```python
from build123d import *

# Parameters (mm, degrees)
CROQUIS1_W              = 41.18
CROQUIS1_H              = 12.95
CROQUIS1_R              = 1.5
SALIENTE_EXTRUIR1_DEPTH = 1
CROQUIS2_W              = 6
CROQUIS2_H              = 7.95
CORTAR_EXTRUIR1_DEPTH   = 0.5


with BuildPart() as part:
    # Croquis1 → Saliente-Extruir1 (new body)
    with BuildSketch(Plane.XY):
        with Locations((-20.59, 6.475)):
            Rectangle(CROQUIS1_W, CROQUIS1_H)
        with Locations((-38.68, 2.5)):
            Circle(CROQUIS1_R, mode=Mode.SUBTRACT)
        with Locations(Location((-38.68, 10.45, 0), (0, 0, 180))):
            Circle(CROQUIS1_R, mode=Mode.SUBTRACT)
        with Locations(Location((-2.5, 2.5, 0), (0, 0, 180))):
            Circle(CROQUIS1_R, mode=Mode.SUBTRACT)
        with Locations((-2.5, 10.45)):
            Circle(CROQUIS1_R, mode=Mode.SUBTRACT)
    extrude(amount=SALIENTE_EXTRUIR1_DEPTH)

    # Croquis2 → Cortar-Extruir1 (cut)
    with BuildSketch(Plane.XY.offset(1)):
        with Locations((-7.5, 6.475)):
            Rectangle(CROQUIS2_W, CROQUIS2_H)
    extrude(amount=-CORTAR_EXTRUIR1_DEPTH, mode=Mode.SUBTRACT)


solid = part.part
```
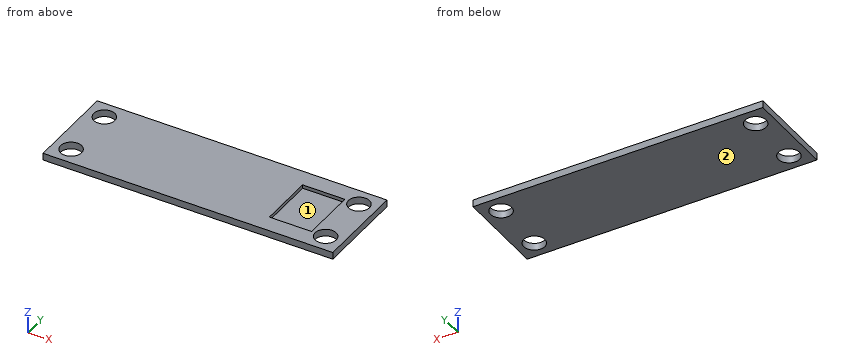
Source: CAD feature listing. Evaluate the final solid. Frame: model axes, mm. Face numbers are marked on the shaded views. Give positions to 0.01 mm unless a question says otherwise; leave off trailing zeros. Order: outer loops, then holes, each group sorted by start corner. A loop starts at its lowest first (then second) coordinate and runs counter-clockwise, first axis right, second up. Notation, with made-up numbers: (75.25, 80.5) -> (120.25, 80.5) arc R23 cw to (120.25, 115.5) -> close; hole circle Ø10 at (20.25, 4). An arc over 180 degrees is marked (long way). Use a Markdown table: item, result.
Q1. Section B-B (x = -2.5). Return the cut outline in (y, z).
A:
| item | result |
|---|---|
| outline | (0, 0) -> (1, 0) -> (1, 1) -> (0, 1) -> close; (4, 0) -> (8.95, 0) -> (8.95, 1) -> (4, 1) -> close; (11.95, 0) -> (12.95, 0) -> (12.95, 1) -> (11.95, 1) -> close |
Q2. Section C-C (y = 8.25). Return the cut outline in (x, z), and give its area (3 significant figures).
A:
| item | result |
|---|---|
| outline | (-41.18, 0) -> (0, 0) -> (0, 1) -> (-4.5, 1) -> (-4.5, 0.5) -> (-10.5, 0.5) -> (-10.5, 1) -> (-41.18, 1) -> close |
| area | 38.2 mm^2 |
Q3. Section D-D (x = -7.5). Return the cut outline in (y, z).
A:
| item | result |
|---|---|
| outline | (0, 0) -> (12.95, 0) -> (12.95, 1) -> (10.45, 1) -> (10.45, 0.5) -> (2.5, 0.5) -> (2.5, 1) -> (0, 1) -> close |
Q4. Material intervals for line 1 (Y direction, x = -2.5, z = 0.6); line 2 (X direction, y = 10.75, z = 0.1); line 3 (Y direction, x = -38, z = 0.3), sorted ascending. Write a range as [from, to].
A:
| item | result |
|---|---|
| line 1 | [0, 1], [4, 8.95], [11.95, 12.95] |
| line 2 | [-41.18, -40.15], [-37.21, -3.97], [-1.03, 0] |
| line 3 | [0, 1.16], [3.84, 9.11], [11.79, 12.95] |
Q5. Section A-A (z = 0.7). Return the cut outline in (x, y), and give its area (3 significant figures).
A:
| item | result |
|---|---|
| outline | (-41.18, 0) -> (0, 0) -> (0, 12.95) -> (-41.18, 12.95) -> close; hole circle Ø3 at (-38.68, 2.5); hole circle Ø3 at (-38.68, 10.45); hole (-10.5, 2.5) -> (-4.5, 2.5) -> (-4.5, 10.45) -> (-10.5, 10.45) -> close; hole circle Ø3 at (-2.5, 2.5); hole circle Ø3 at (-2.5, 10.45) |
| area | 457 mm^2 |
Q6. First-contact query: P1, Ø4, axis at x = -38.68, y = 10.45, coming from the -Z side; P2, Ø1.8, axis at x = -38.68, y = 2.5, coming from the +Z side. Flat tips, straight axial feed; report the tip coordinate or a pass-through.
A:
| item | result |
|---|---|
| P1 | z = 0 |
| P2 | through |
Q7. Pull-direction query (X, two-part tool) for the marked faces 1 and 2; classes: +X half, -X half, draft (parallel to the pull), parting line (faces both ways), or undercut.
A:
| item | result |
|---|---|
| face 1 | undercut |
| face 2 | draft |
